Source: CAD feature listing. Evaluate the final solid. Frame: model axes, mm. Face numbers are marked on the shaded views. A direction names the side the tool comes from. Give positions to 0.01 mm unless a question says otherwise; leave off trailing zeros. Order: outer loops, then holes, each group sorted by start corner. A loop starts at its lowest first (then second) coordinate and runs counter-clockwise, first axis right, second up. Notation, with made-up numbers: M 34,70.5 L 65,70.5 A8 ccw 65,79.5 Z; hole C 64.5,-27 d11. An arc over 180 degrees is marked long. Return JSON: item names as keys, results as strings.
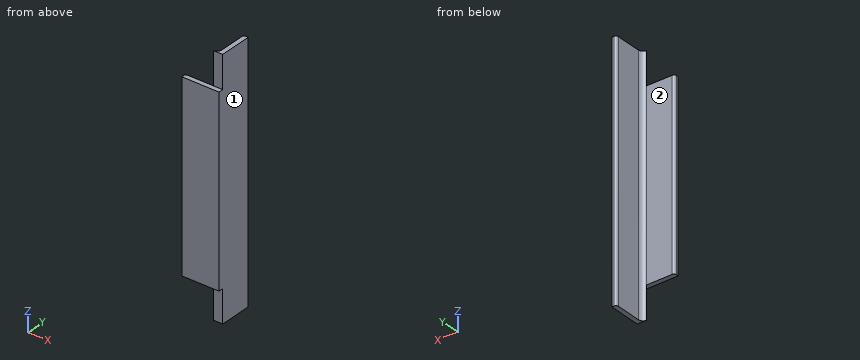
from build123d import *

# Parameters (mm, degrees)
BOSS_EXTRUDE1_DEPTH = 609.6
SKETCH3_W           = 1049.2
SKETCH3_H           = 25.4
CUT_EXTRUDE2_DEPTH  = 30.48
SKETCH6_W           = 25.4
SKETCH6_H           = 3.175
CUT_EXTRUDE4_DEPTH  = 22.23
SKETCH7_W           = 25.4
SKETCH7_H           = 3.175
CUT_EXTRUDE5_DEPTH  = 22.23


with BuildPart() as part:
    # Sketch2 → Boss-Extrude1 (new, symmetric)
    with BuildSketch(Plane.XY):
        with BuildLine():
            Line((-12.7, -12.7), (12.7, -12.7))
            Line((12.7, -12.7), (12.7, 12.7))
            Line((12.7, 12.7), (11.1125, 12.7))
            ThreePointArc((11.1125, 12.7), (9.989967985, 12.235032015), (9.525, 11.1125))
            Line((9.525, 11.1125), (9.525, -6.35))
            ThreePointArc((9.525, -6.35), (8.59506403, -8.59506403), (6.35, -9.525))
            Line((6.35, -9.525), (-11.1125, -9.525))
            ThreePointArc((-11.1125, -9.525), (-12.235032015, -9.989967985), (-12.7, -11.1125))
            Line((-12.7, -11.1125), (-12.7, -12.7))
        make_face()
    extrude(amount=BOSS_EXTRUDE1_DEPTH, both=True)

    # Sketch3 → Cut-Extrude2 (cut)
    with BuildSketch(Plane(origin=(12.7, 0, 0), x_dir=(0, 0, -1), z_dir=(1, 0, 0))):
        with Locations((85, 0)):
            Rectangle(SKETCH3_W, SKETCH3_H)
    extrude(amount=-CUT_EXTRUDE2_DEPTH, mode=Mode.SUBTRACT)

    # Sketch6 → Cut-Extrude4 (cut)
    with BuildSketch(Plane(origin=(0, 0, 439.6), x_dir=(-1, 0, 0), z_dir=(0, 0, -1))):
        with Locations((0, -11.1125)):
            Rectangle(SKETCH6_W, SKETCH6_H)
    extrude(amount=-CUT_EXTRUDE4_DEPTH, mode=Mode.SUBTRACT)

    # Sketch7 → Cut-Extrude5 (cut)
    with BuildSketch(Plane.XY.offset(609.6)):
        with Locations((0, -11.1125)):
            Rectangle(SKETCH7_W, SKETCH7_H)
    extrude(amount=-CUT_EXTRUDE5_DEPTH, mode=Mode.SUBTRACT)


solid = part.part
1. Set-up query: the marked faces 1 and 2. Return all of +Z, -Z, +X, -X, +Y, -Y with unobstructed straight access to the full face (end or side cutting, diameter ignored); none if empty.
Evaluation:
{"face 1": "+Z, -Z, +X, +Y, -Y", "face 2": "+Z, -Z, -X, +Y"}
2. First-contact query: pin 1 (14 mm diameter, centred on x = -3.5, z = 510, fed in from +Y) (3 decimals); pin 2 (7 mm diameter, centred on x = 10, z = 603, fed in from -Y) (3 decimals); pin 3 (3.5 mm diameter, centred on x = 0, y = -12, fed in from -Z). Flat tips, straight axial feed; report the tip coordinate or a pass-through.
Evaluation:
{"pin 1": "stops at y = -9.525", "pin 2": "stops at y = -9.525", "pin 3": "stops at z = 461.83"}
3. Ray query, probe 1 along Y at (x, z) = (1.5, 470.5) (3 decimals); probe 2 along X at (y, z) = (11.25, 585.5); probe 3 along Y at (x, z) = (8.75, 503). Return the intervals inside material, ascending.
Evaluation:
{"probe 1": "y = -12.7 to -9.525", "probe 2": "x = 9.53 to 12.7", "probe 3": "y = -12.7 to -8.43"}
4. Section query B-B (x = -9.25). Return loops of the section in (y, z) (3 decimals).
Evaluation:
{"outline": "M -12.7,461.83 L -9.525,461.83 L -9.525,587.37 L -12.7,587.37 Z"}
5. Section query C-C (y = -0.75). Return loops of the section in (x, z) (3 decimals).
Evaluation:
{"outline": "M 9.525,439.6 L 12.7,439.6 L 12.7,609.6 L 9.525,609.6 Z"}
